Part model, mm, in its own coordinate system. Face numbers are marked on the shaded views. A direction names the side the tool comes from. Round coordinates to 2 decimals unless told otherwise and drop trailing zeros. Write each loop counter-clockwise with the first axis right and the second up, starting at its lowest first coordinate (ties: lowest second). Pieces come first, ordered by that corner, then holes.
Autodesk Inventor part; units mm, degrees
ref_plane "YZ Plane" through (0, 0, 0) normal (1, 0, 0) x (0, 1, 0)
ref_plane "XZ Plane" through (0, 0, 0) normal (0, 1, 0) x (-1, 0, 0)
ref_plane "XY Plane" through (0, 0, 0) normal (0, 0, 1) x (1, 0, 0)
sketch "Skizze1" plane through (0, 0, 0) normal (0, 1, 0) x (-1, 0, 0)
  line L0 (10, 10) -> (-10, 10)
  line L1 (-10, 10) -> (-10, -10)
  line L2 (-10, -10) -> (10, -10)
  line L3 (10, -10) -> (10, 10)
  line L4 (10, 10) -> (-10, -10) construction
  line L5 (-10, 10) -> (10, -10) construction
  point P0 (0, 0)
  dimension "d0" = 20
  dimension "d1" = 20
extrude "Extrusion1" add sketch "Skizze1" along normal blind 34.5
sketch "Skizze2" plane through (0, 0, 0) normal (0, -1, 0) x (1, 0, 0)
  line L0 (-8.9654, -8) -> (-1.6431, -8)
  line L1 (8, 1.6431) -> (8, 9.2)
  line L2 (-10, 10) -> (10, 10)
  line L3 (-10, -10) -> (-10, 10)
  line L4 (8, 10) -> (-10, 10)
  line L5 (-10, 10) -> (-10, -8)
  line L6 (-10, -8) -> (8, -8)
  line L7 (8, -8) -> (8, 10)
  line L8 (10, 10) -> (10, -10)
  line L9 (-10, 10) -> (10, 10)
  line L10 (-10, -10) -> (-10, 10)
  line L11 (10, -10) -> (-10, -10)
  circle A0 centre (-1.6431, 1.6431) radius 9.6431
  point P0 (0, 0)
extrude "Extrusion2" cut sketch "Skizze2" against normal through all contours L0 L6 L7 L1 L2 L8 L11 L3 | A0 L7 L6
sketch "Skizze3" plane through (0, 34.5, 0) normal (0, 1, 0) x (1, 0, 0)
  line L0 (0.9, -9.6) -> (0.9, -12.8936)
  line L1 (0.9, -12.8936) -> (1.9, -12.8936)
  line L2 (1.9, -12.8936) -> (2.4, -11.85)
  line L3 (2.4, -11.85) -> (1.9, -11.85)
  line L4 (1.9, -12.8936) -> (1.9, -9.6)
  line L5 (-2.9, -12.8936) -> (-2.9, -9.6)
  line L6 (-3.9, -9.6) -> (-3.9, -12.8936)
  line L7 (-3.9, -11.85) -> (-4.4, -11.85)
  line L8 (-4.4, -11.85) -> (-3.9, -12.8936)
  line L9 (-3.9, -12.8936) -> (-2.9, -12.8936)
  line L10 (0.9, -12.8936) -> (1.9, -12.8936)
  line L11 (1.9, -12.8936) -> (1.9, -9.6)
  line L12 (1.9, -9.6) -> (0.9, -9.6)
  line L13 (0.9, -9.6) -> (0.9, -12.8936)
  line L14 (-2.9, -12.8936) -> (-3.9, -12.8936)
  line L15 (-3.9, -12.8936) -> (-3.9, -9.6)
  line L16 (-3.9, -9.6) -> (-2.9, -9.6)
  line L17 (-2.9, -9.6) -> (-2.9, -12.8936)
  point P0 (0, 0)
extrude "Extrusion3" add sketch "Skizze3" against normal up to surface (34.5 mm away)
sketch "Skizze6" plane through (0, 34.5, 0) normal (0, 1, 0) x (1, 0, 0)
  line L0 (-7, -11.6) -> (5, -11.6)
  line L1 (5, -11.6) -> (5, -8.4)
  line L2 (5, -8.4) -> (-7, -8.4)
  line L3 (-7, -8.4) -> (-7, -11.6)
  line L4 (-2.9, -10) -> (0.9, -10)
  line L5 (-7, -11.6) -> (5, -8.4) construction
  line L6 (5, -11.6) -> (-7, -8.4) construction
  line L7 (-10, 8) -> (-10, -10)
  line L8 (-10, -10) -> (8, -10)
  line L9 (8, -10) -> (8, 8)
  line L10 (8, 8) -> (-10, 8)
  line L11 (-10, 8) -> (-10, -10)
  point P0 (0, 0)
  point P1 (-1, -10)
  point P2 (5, -10)
  point P3 (-7, -10)
  dimension "d26" = 12
  dimension "d27" = 3.2
extrude "Extrusion6" cut sketch "Skizze6" against normal through all both and the other way through all contours L8 L7 L10 L9 L1 L2 L3
move faces "Verschieben2" translate (0, -26.5, 0) faces at (-0.3667, 34.5, 8.9333)
fillet "Rundung5" radius 1.5 2 edges at (5, 4, 8.4) (-7, 4, 8.4)
properties part number "CableClip"
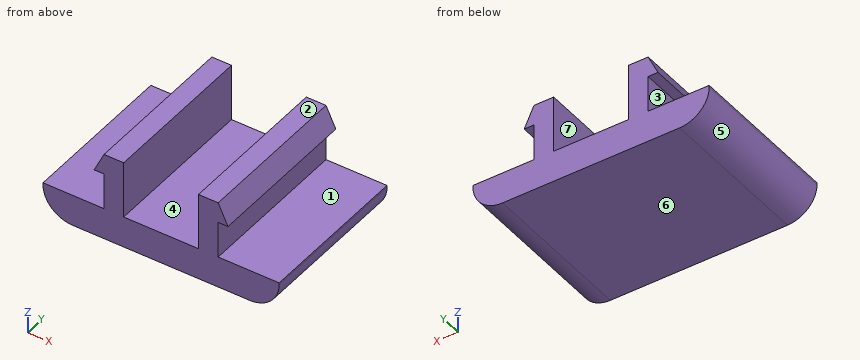
Q1. Mould opens along X. For the marked faces 5, 6 and 7 say: +X half, -X half, draft (parallel to the pull), parting line (faces both ways), or undercut.
Values follow:
face 5: -X half
face 6: draft
face 7: undercut
Q2. Wall check: L1, parallel to X at y = 2, z = 11.5; L2, parallel to Z at x = -5.25, y = 0.5; L3, parallel to X at y = 6, z = 12.55. Give the ranges that are in metal, low to high.
Values follow:
L1: x = -3.9 to -2.9, 0.9 to 1.9
L2: z = 8.4 to 10
L3: x = -4.06 to -2.9, 0.9 to 2.06
Q3. Drop flat-ended pins along their axis: pin 1 (0.6 mm diameter, centred on y = 4, z = 11, fed in from -X); pin 2 (0.9 mm diameter, centred on y = 4, z = 11.5, fed in from -X); pin 3 (1.6 mm diameter, centred on x = -5.5, y = 4, fed in from +Z). Give the stop position or say it passes through.
Values follow:
pin 1: stops at x = -3.9
pin 2: stops at x = -4.4
pin 3: stops at z = 10
Q4. Which spindle directions (+Z, -Z, +X, -X, +Y, -Y) get a long thin tool onto all of the face, cutting with end or side? Do the marked faces 1, 2, 3 and 4. Say none if no direction does.
Values follow:
face 1: +X, +Y, -Y
face 2: +Z, +X, -X, +Y, -Y
face 3: -X, +Y, -Y
face 4: +Z, +Y, -Y
Q5. Cut at D-D on z = 12.5. Write the cut outline in (x, y).
Values follow:
outline: (-4.09, 0) - (-2.9, 0) - (-2.9, 8) - (-4.09, 8) - close; (0.9, 0) - (2.09, 0) - (2.09, 8) - (0.9, 8) - close
Q6. Cut at B-B on y = 5. Write the cut outline in (x, z), plus the area to 3 significant figures.
Values follow:
outline: (-7, 9.9) arc R1.5 ccw to (-5.5, 8.4) - (3.5, 8.4) arc R1.5 ccw to (5, 9.9) - (5, 10) - (1.9, 10) - (1.9, 11.85) - (2.4, 11.85) - (1.9, 12.89) - (0.9, 12.89) - (0.9, 10) - (-2.9, 10) - (-2.9, 12.89) - (-3.9, 12.89) - (-4.4, 11.85) - (-3.9, 11.85) - (-3.9, 10) - (-7, 10) - close
area: 24.5 mm2
Q7. Cut at A-A on z = 11. Write the cut outline in (x, y), plus the area to 3 significant figures.
Values follow:
outline: (-3.9, 0) - (-2.9, 0) - (-2.9, 8) - (-3.9, 8) - close; (0.9, 0) - (1.9, 0) - (1.9, 8) - (0.9, 8) - close
area: 16.0 mm2
Q8. Cut at C-C on x = -4.75. Write the cut outline in (y, z), plus the area to 3 significant figures.
Values follow:
outline: (0, 8.4) - (8, 8.4) - (8, 10) - (0, 10) - close
area: 12.8 mm2
